Autodesk Inventor part; units mm, degrees
ref_plane "YZ Plane" through (0, 0, 0) normal (1, 0, 0) x (0, 1, 0)
ref_plane "XZ Plane" through (0, 0, 0) normal (0, 1, 0) x (-1, 0, 0)
ref_plane "XY Plane" through (0, 0, 0) normal (0, 0, 1) x (1, 0, 0)
sketch "Sketch1" plane through (0, 0, 0) normal (0, 1, 0) x (-1, 0, 0)
  circle A0 centre (0, 0) radius 22
  dimension "d0" = 44
extrude "Extrusion1" add sketch "Sketch1" along normal blind 7
sketch "Sketch3" plane through (0, 0, 0) normal (0, -1, 0) x (1, 0, 0)
  circle A0 centre (0, 0) radius 15
  dimension "d4" = 30
extrude "Extrusion2" [suppressed]
sketch "Sketch4" plane through (0, 2, 0) normal (0, -1, 0) x (1, 0, 0)
  circle A0 centre (0, 0) radius 12
  dimension "d11" = 24
extrude "Extrusion3" [suppressed]
sketch "Sketch5" plane through (0, 4, 0) normal (0, -1, 0) x (1, 0, 0)
  circle A0 centre (0, 0) radius 10
  dimension "d14" = 20
extrude "Extrusion4" [suppressed]
sketch "Sketch6" plane through (0, 6, 0) normal (0, -1, 0) x (1, 0, 0)
  circle A0 centre (0, 0) radius 8.5
  dimension "d17" = 17
extrude "Extrusion5" [suppressed]
sketch "Sketch7" plane through (0, 8, 0) normal (0, -1, 0) x (1, 0, 0)
  circle A0 centre (0, 0) radius 7
  dimension "d20" = 14
extrude "Extrusion6" [suppressed]
sketch "Sketch9" plane through (0, 7, 0) normal (0, 1, 0) x (1, 0, 0)
  line L0 (20, 8) -> (7, 8)
  line L1 (7, 8) -> (7, -8)
  line L2 (7, -8) -> (20, -8)
  line L3 (20, -8) -> (20, 8)
  line L4 (-20, 8) -> (-7, 8)
  line L5 (-7, 8) -> (-7, -8)
  line L6 (-7, -8) -> (-20, -8)
  line L7 (-20, -8) -> (-20, 8)
  line L8 (18, 6) -> (9, 6)
  line L9 (9, 6) -> (9, -6)
  line L10 (9, -6) -> (18, -6)
  line L11 (18, -6) -> (18, 6)
  line L12 (-9, 6) -> (-18, 6)
  line L13 (-18, 6) -> (-18, -6)
  line L14 (-18, -6) -> (-9, -6)
  line L15 (-9, -6) -> (-9, 6)
  point P0 (0, 0)
  point P1 (7, 0)
  point P2 (-7, 0)
  point P3 (9, 0)
  point P4 (-9, 0)
  dimension "d29" = 13
  dimension "d30" = 16
  dimension "d31" = 7
  dimension "d32" = 13
  dimension "d33" = 16
  dimension "d34" = 7
  dimension "d35" = 9
  dimension "d36" = 12
  dimension "d37" = 2
  dimension "d38" = 9
  dimension "d39" = 12
  dimension "d40" = 2
extrude "Extrusion8" add sketch "Sketch9" along normal blind 20
sketch "Sketch8" plane through (0, 0, 0) normal (0, -1, 0) x (1, 0, 0)
  circle A0 centre (0, 19) radius 1.25
  circle A1 centre (0, -19) radius 1.25
  point P0 (0, 0)
  dimension "d23" = 2.5
  dimension "d24" = 2.5
  dimension "d25" = 19
  dimension "d26" = 19
extrude "Extrusion7" cut sketch "Sketch8" against normal blind 14
sketch "Sketch10" plane through (-7, 10, 0) normal (1, 0, 0) x (0, 0, -1)
  circle A0 centre (0, 2) radius 3
  line L0 (-8, 17) -> (8, 17)
  point P0 (0, -10)
  dimension "d43" = 6
  dimension "d44" = 15
extrude "Extrusion9" cut sketch "Sketch10" against normal blind 2
sketch "Sketch11" plane through (7, 7, -8) normal (-1, 0, 0) x (0, 0, 1)
  circle A0 centre (8, 5) radius 2
  line L0 (0, 20) -> (16, 20)
  point P0 (8, -7)
  dimension "d47" = 4
  dimension "d48" = 15
extrude "Extrusion10" cut sketch "Sketch11" against normal blind 2
sketch "Sketch12" plane through (0, 0, 0) normal (1, 0, 0) x (0, 1, 0)
  line L0 (7, 6.5) -> (0, 17)
  line L1 (7, 0) -> (7, 6.5)
  line L2 (7, 0) -> (0, 0)
  line L3 (0, 0) -> (0, 17)
  line L4 (0, 22) -> (0, -22)
  dimension "d54" = 6.5
  dimension "d55" = 17
  dimension "d56" = 7
revolve "Revolution1" cut sketch "Sketch12" angle 360 about axis through (0, 7, 0) along (0, -1, 0)
properties part number "funil"
Check sheet for the modelled part. Datum: model origin and axes. Units: mm. A direction names the side the tool comes from. Coordinates: 2 decimals unless noted, no trailing zeros. Order: outer loops, then holes, each group sorted by start corner. A loop starts at its lowest first (then second) coordinate and runs counter-clockwise, first axis right, second up. Notation, with made-up numbers: (67.5, 56.25) -> (81.5, 56.25) arc R27 ccw to (81.5, 79.25) -> close; hole circle Ø2 at (-31, 23). An arc over 180 degrees is marked (long way). Write item = value, one per line. Start each with the question number.
1) Cross-section at D-D (x = 0). Enter the section's corners in (y, z), then the cut area to 4 significant figures.
2) Mould release check, pull along Z, two halves, no side actions. Record for faces 5 (the flat face through (-14, 17, -8)), 6 (the flat face through (-13, 17, -6)), 7 (the flat face through (-5, 7, 5)): +Z half, -Z half, draft (parallel to the pull), parting line (faces both ways), or undercut.
3) Cross-section at B-B (y = 12). Enter the section's corners in (x, z).
4) Cross-section at A-A (y = 24.25). Enter the section's corners in (x, z).
5) Access from +Z, -Z, +X, -X, +Y, -Y to the whole of each face (thin tool, end or side, straight path). Record for faces 1 (the flat face through (14, 17, -6)), 2 (the flat face through (13, 17, 8)), 3 (the flat face through (14, 17, -8)), 4 (the flat face through (20, 17, 0)).
6) Go/stop test with flat-tipped pins: P1, Ø12, axis at y = 5.5, z = 14, coming from the -X side; P2, Ø5, axis at y = 13.5, z = -3.5, coming from the -X side; P3, Ø5, axis at x = 14, y = 17.5, coming from the -Z side; P4, Ø1, axis at y = 18.5, z = -10, coming from the -X side. Record where each tip stops, or that it passes through.
7) Cross-section at C-C (z = 0). State how many separate pieces and enclosed holes the cut face has, then the cut area to 4 significant figures.
8) Material ranges on L1, parallel to X at y = 23.5, z = 1; L2, parallel to Z at x = 0, y = 3.75 (3 decimals); L3, parallel to X at y = 16.5, z = -6.5, recorded low to high.
Ans:
q1.outline = (0, -22) -> (7, -22) -> (7, -20.25) -> (0, -20.25) -> close; (0, -17.75) -> (7, -17.75) -> (7, -6.5) -> (0, -17) -> close; (0, 17) -> (7, 6.5) -> (7, 17.75) -> (0, 17.75) -> close; (0, 20.25) -> (7, 20.25) -> (7, 22) -> (0, 22) -> close
q1.area = 108.5 mm²
q2.face_5 = -Z half
q2.face_6 = undercut
q2.face_7 = draft
q3.outline = (-20, -8) -> (-7, -8) -> (-7, -3) -> (-9, -3) -> (-9, -6) -> (-18, -6) -> (-18, 6) -> (-9, 6) -> (-9, 3) -> (-7, 3) -> (-7, 8) -> (-20, 8) -> close; (7, -8) -> (20, -8) -> (20, 8) -> (7, 8) -> (7, 2) -> (9, 2) -> (9, 6) -> (18, 6) -> (18, -6) -> (9, -6) -> (9, -2) -> (7, -2) -> close
q4.outline = (-20, -8) -> (-7, -8) -> (-7, 8) -> (-20, 8) -> close; (7, -8) -> (20, -8) -> (20, 8) -> (7, 8) -> close; hole (-18, -6) -> (-9, -6) -> (-9, 6) -> (-18, 6) -> close; hole (9, -6) -> (18, -6) -> (18, 6) -> (9, 6) -> close
q5.face_1 = +Y
q5.face_2 = +Z, +X, -X, +Y
q5.face_3 = -Z, +X, -X, +Y
q5.face_4 = +Z, -Z, +X, +Y
q6.P1 = -20.49
q6.P2 = -20
q6.P3 = -8
q6.P4 = through
q7.separate_pieces = 4
q7.enclosed_holes = 0
q7.area = 283.5 mm²
q8.L1 = -20 to -18, -9 to -7, 7 to 9, 18 to 20
q8.L2 = -22 to -20.25, -17.75 to -11.375, 11.375 to 17.75, 20.25 to 22
q8.L3 = -20 to -7, 7 to 20
